```python
from build123d import *

# Parameters (mm, degrees)
F0_W     = 77
F0_H     = 37
F0_W_2   = 73
F0_H_2   = 33
F1_DEPTH = 500
F3_DEPTH = 128.275266
F5_DEPTH = 87.845365


with BuildPart() as f1:
    # F0 (on Front) → F1 (new body)
    with BuildSketch(Plane.XZ):
        with Locations((38.5, -18.5)):
            Rectangle(F0_W, F0_H)
        with Locations((38.5, -18.5)):
            Rectangle(F0_W_2, F0_H_2, mode=Mode.SUBTRACT)
    extrude(amount=F1_DEPTH)

    # F2 (on face) → F3 (cut)
    with BuildSketch(Plane(origin=(0, 0, 0), x_dir=(0, -1, 0), z_dir=(-1, 0, 0))):
        Polygon((36.537793, 0), (0, 0), (0, -37), align=None)
    extrude(amount=-F3_DEPTH, mode=Mode.SUBTRACT)

    # F4 (on face) → F5 (cut)
    with BuildSketch(Plane.YZ.offset(77)):
        Polygon((-463, 0), (-500, 0), (-500, -37), align=None)
    extrude(amount=-F5_DEPTH, mode=Mode.SUBTRACT)


solid = f1.part
```
Work out the finished part from the listing and answer in its coordinate system (mm). A direction names the side the tool comes from. Give positions to 0.01 mm unless a question says otherwise; leave off trailing zeros. Loops run counter-clockwise (first coordinate to the right, second up) from the corner with the lowest first, then second, coordinate; pieces in that order, holes last. Notation, with made-up numbers: (-0.5, 61.25) -> (19.5, 61.25) arc R30 cw to (19.5, 91.25) -> close; hole circle Ø4 at (54.25, 86.5). An arc over 180 degrees is marked (long way). Put each result on its own line as item: value. Start each with the question number.
Item 1: The part is cut by section A-A (y = -103.5). Give the vertices of the cut face in (x, z).
Item 2: The mould has two halves that part along X. Classify faces 3 (the face through (77, -246, -19)), 4 (the face through (2, -247, -19)), 5 (the face through (38, -246, -37)), 6 (the face through (38, -247, -35)): released by +X, released by -X, zero draft, split by the parting line, or undercut.
Item 3: Find the intervals of material crossed by L1, parallel to Z at x = 38, y = -98; L2, parallel to X at y = -155.5, z = -18, in increasing order. Write a range as [from, to].
Item 4: The part is cut by section B-B (x = 57). Give the vertices of the cut face in (y, z).
Item 5: The part is cut by section C-C (z = -9.5). Give the vertices of the cut face in (x, y), then the cut area to 3 significant figures.
Item 6: Which of the six approach directions +Z, -Z, +X, -X, +Y, -Y give full straight-line access (tool end or side, diameter ignored) to faces 1 (the face through (38, -247, 0)), 2 (the face through (75, -247, -19))?
Answers below:
1. outline: (0, -37) -> (77, -37) -> (77, 0) -> (0, 0) -> close; hole (2, -35) -> (75, -35) -> (75, -2) -> (2, -2) -> close
2. face 3: released by +X
2. face 4: undercut
2. face 5: zero draft
2. face 6: undercut
3. L1: [-37, -35], [-2, 0]
3. L2: [0, 2], [75, 77]
4. outline: (-500, -37) -> (0, -37) -> (-1.98, -35) -> (-498, -35) -> close; (-465, -2) -> (-34.56, -2) -> (-36.54, 0) -> (-463, 0) -> close
5. outline: (0, -472.5) -> (2, -472.5) -> (2, -27.16) -> (0, -27.16) -> close; (75, -472.5) -> (77, -472.5) -> (77, -27.16) -> (75, -27.16) -> close
5. area: 1,780 mm2
6. face 1: +Z, +X, -X, +Y, -Y
6. face 2: +Y, -Y
